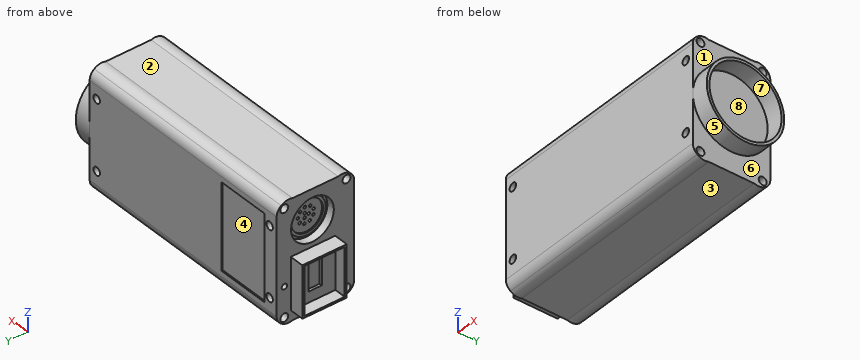
from build123d import *

# Parameters (mm, degrees)
SALIENTE_EXTRUIR2_DEPTH = 86.7
CROQUIS4_R              = 1.5
CORTAR_EXTRUIR1_DEPTH   = 4
CROQUIS5_R              = 14.5
CROQUIS5_R_2            = 13.5
SALIENTE_EXTRUIR3_DEPTH = 6.45
CROQUIS6_R              = 1.5
CORTAR_EXTRUIR2_DEPTH   = 3.5
CROQUIS8_W              = 20
CROQUIS8_H              = 32
CORTAR_EXTRUIR3_DEPTH   = 0.5
CROQUIS10_R             = 1
CORTAR_EXTRUIR6_DEPTH   = 4.5
CORTAR_EXTRUIR7_START   = -4.5
CROQUIS11_R             = 1.5
CORTAR_EXTRUIR7_DEPTH   = 4.5
CROQUIS12_W             = 19.288477202
CROQUIS12_H             = 16.6
SALIENTE_EXTRUIR4_DEPTH = 5.35
CROQUIS13_W             = 18
CROQUIS13_H             = 15.1
CORTAR_EXTRUIR8_DEPTH   = 4.35
CROQUIS14_W             = 10
CROQUIS14_H             = 5
CORTAR_EXTRUIR9_DEPTH   = 1
CROQUIS15_R             = 8
CORTAR_EXTRUIR10_DEPTH  = 3
CROQUIS16_R             = 7
CROQUIS16_R_2           = 6
SALIENTE_EXTRUIR5_DEPTH = 0.5
CROQUIS17_R             = 0.5
CORTAR_EXTRUIR12_DEPTH  = 1.5
CROQUIS18_R             = 1.5
CORTAR_EXTRUIR13_DEPTH  = 3.5


with BuildPart() as part:
    # Croquis3 → Saliente-Extruir2 (new body)
    with BuildSketch(Plane(origin=(0, 0, 0), x_dir=(0, 0, -1), z_dir=(1, 0, 0))):
        with BuildLine():
            Line((4, 0), (40, 0))
            ThreePointArc((40, 0), (41.842910618, 0.449833743), (43.271319545, 1.698159773))
            ThreePointArc((43.271319545, 1.698159773), (44.186191252, 3.744879364), (44, 5.979019946))
            Line((44, 5.979019946), (44, 23.020980054))
            ThreePointArc((44, 23.020980054), (44.186191252, 25.255120636), (43.271319545, 27.301840227))
            ThreePointArc((43.271319545, 27.301840227), (41.842910618, 28.550166257), (40, 29))
            Line((40, 29), (4, 29))
            ThreePointArc((4, 29), (2.157089382, 28.550166257), (0.728680455, 27.301840227))
            ThreePointArc((0.728680455, 27.301840227), (-0.186191252, 25.255120636), (0, 23.020980054))
            Line((0, 23.020980054), (0, 5.979019946))
            ThreePointArc((0, 5.979019946), (-0.186191252, 3.744879364), (0.728680455, 1.698159773))
            ThreePointArc((0.728680455, 1.698159773), (2.157089382, 0.449833743), (4, 0))
        make_face()
    extrude(amount=SALIENTE_EXTRUIR2_DEPTH)

    # Croquis4 → Cortar-Extruir1 (cut)
    with BuildSketch(Plane(origin=(86.7, 0, 0), x_dir=(0, 0, -1), z_dir=(1, 0, 0))):
        with Locations((2.364340227, 26.150920114)):
            Circle(CROQUIS4_R)
        with Locations(Location((41.635659773, 26.150920114, 0), (0, 0, 180))):
            Circle(CROQUIS4_R)
        with Locations((41.635659773, 2.849079886)):
            Circle(CROQUIS4_R)
        with Locations(Location((2.364340227, 2.849079886, 0), (0, 0, 180))):
            Circle(CROQUIS4_R)
    extrude(amount=-CORTAR_EXTRUIR1_DEPTH, mode=Mode.SUBTRACT)

    # Croquis5 → Saliente-Extruir3 (add)
    with BuildSketch(Plane(origin=(86.7, 0, 0), x_dir=(0, 0, -1), z_dir=(1, 0, 0))):
        with Locations(Location((22, 14.5, 0), (0, 0, 270))):
            Circle(CROQUIS5_R)
        with Locations(Location((22, 14.5, 0), (0, 0, 180))):
            Circle(CROQUIS5_R_2, mode=Mode.SUBTRACT)
    extrude(amount=SALIENTE_EXTRUIR3_DEPTH)

    # Croquis6 → Cortar-Extruir2 (cut)
    with BuildSketch(Plane(origin=(0, 29, 0), x_dir=(1, 0, 0), z_dir=(0, 1, 0))):
        with Locations(Location((83.45, 35, 0), (0, 0, 270))):
            Circle(CROQUIS6_R)
        with Locations(Location((83.45, 9, 0), (0, 0, 270))):
            Circle(CROQUIS6_R)
        with Locations(Location((3.25, 9, 0), (0, 0, 90))):
            Circle(CROQUIS6_R)
        with Locations(Location((3.25, 35, 0), (0, 0, 90))):
            Circle(CROQUIS6_R)
    extrude(amount=-CORTAR_EXTRUIR2_DEPTH, mode=Mode.SUBTRACT)

    # Croquis8 → Cortar-Extruir3 (cut)
    with BuildSketch(Plane(origin=(0, 29, 0), x_dir=(1, 0, 0), z_dir=(0, 1, 0))):
        with Locations((15.654947335, 22)):
            Rectangle(CROQUIS8_W, CROQUIS8_H)
    extrude(amount=-CORTAR_EXTRUIR3_DEPTH, mode=Mode.SUBTRACT)

    # Croquis10 → Cortar-Extruir6 (cut)
    with BuildSketch(Plane.ZY):
        with Locations((-30.5, 6.1)):
            Circle(CROQUIS10_R)
        with Locations((-30.5, 26.1)):
            Circle(CROQUIS10_R)
    extrude(amount=-CORTAR_EXTRUIR6_DEPTH, mode=Mode.SUBTRACT)

    # Croquis11 → Cortar-Extruir7 (cut)
    with BuildSketch(Plane.ZY.offset(CORTAR_EXTRUIR7_START)):
        with Locations((-41.635659773, 26.150920114)):
            Circle(CROQUIS11_R)
        with Locations(Location((-41.635659773, 2.849079886, 0), (0, 0, 180))):
            Circle(CROQUIS11_R)
        with Locations((-2.364340227, 2.849079886)):
            Circle(CROQUIS11_R)
        with Locations(Location((-2.364340227, 26.150920114, 0), (0, 0, 180))):
            Circle(CROQUIS11_R)
    extrude(amount=CORTAR_EXTRUIR7_DEPTH, mode=Mode.SUBTRACT)

    # Croquis12 → Saliente-Extruir4 (add)
    with BuildSketch(Plane.ZY):
        with Locations((-30.5, 15.4)):
            Rectangle(CROQUIS12_W, CROQUIS12_H)
    extrude(amount=SALIENTE_EXTRUIR4_DEPTH)

    # Croquis13 → Cortar-Extruir8 (cut)
    with BuildSketch(Plane.ZY.offset(5.35)):
        with Locations((-30.489294878, 15.4)):
            Rectangle(CROQUIS13_W, CROQUIS13_H)
    extrude(amount=-CORTAR_EXTRUIR8_DEPTH, mode=Mode.SUBTRACT)

    # Croquis14 → Cortar-Extruir9 (cut)
    with BuildSketch(Plane.ZY.offset(1)):
        with Locations((-30.5, 15.4)):
            Rectangle(CROQUIS14_W, CROQUIS14_H)
    extrude(amount=-CORTAR_EXTRUIR9_DEPTH, mode=Mode.SUBTRACT)

    # Croquis15 → Cortar-Extruir10 (cut)
    with BuildSketch(Plane.ZY):
        with Locations((-11.119013901, 15.6)):
            Circle(CROQUIS15_R)
    extrude(amount=-CORTAR_EXTRUIR10_DEPTH, mode=Mode.SUBTRACT)

    # Croquis16 → Saliente-Extruir5 (add)
    with BuildSketch(Plane.ZY.offset(-3)):
        with Locations((-11.119013901, 15.6)):
            Circle(CROQUIS16_R)
        with Locations((-11.119013901, 15.6)):
            Circle(CROQUIS16_R_2, mode=Mode.SUBTRACT)
    extrude(amount=SALIENTE_EXTRUIR5_DEPTH)

    # Croquis17 → Cortar-Extruir12 (cut)
    with BuildSketch(Plane.ZY.offset(-3)):
        with Locations((-11.025814876, 18.6)):
            Circle(CROQUIS17_R)
        with Locations((-9.119256477, 17.838226151)):
            Circle(CROQUIS17_R)
        with Locations((-8.148406801, 16.029161411)):
            Circle(CROQUIS17_R)
        with Locations((-8.567537202, 14.019287277)):
            Circle(CROQUIS17_R)
        with Locations((-10.180531906, 12.749046194)):
            Circle(CROQUIS17_R)
        with Locations((-12.232652766, 12.812798081)):
            Circle(CROQUIS17_R)
        with Locations((-13.763689624, 14.180712723)):
            Circle(CROQUIS17_R)
        with Locations((-14.057253319, 16.212727655)):
            Circle(CROQUIS17_R)
        with Locations((-12.975982135, 17.958040507)):
            Circle(CROQUIS17_R)
        with Locations((-11.985039305, 16.1)):
            Circle(CROQUIS17_R)
        with Locations((-10.252988497, 16.1)):
            Circle(CROQUIS17_R)
        with Locations((-11.119013901, 14.6)):
            Circle(CROQUIS17_R)
    extrude(amount=-CORTAR_EXTRUIR12_DEPTH, mode=Mode.SUBTRACT)

    # Croquis18 → Cortar-Extruir13 (cut)
    with BuildSketch(Plane.XZ):
        with Locations(Location((83.45, -8.377668185, 0), (0, 0, 270))):
            Circle(CROQUIS18_R)
        with Locations(Location((83.45, -34.377668185, 0), (0, 0, 270))):
            Circle(CROQUIS18_R)
        with Locations(Location((3.25, -34.377668185, 0), (0, 0, 90))):
            Circle(CROQUIS18_R)
        with Locations(Location((3.25, -8.377668185, 0), (0, 0, 90))):
            Circle(CROQUIS18_R)
    extrude(amount=-CORTAR_EXTRUIR13_DEPTH, mode=Mode.SUBTRACT)


solid = part.part
The listing builds one solid part. Answer for the finished solid, in the listing's coordinates (mm). Face numbers are marked on the shaded views. A direction names the side the tool comes from. Give positions to 0.01 mm unless a question says otherwise; leave off trailing zeros. Order: outer loops, then holes, each group sorted by start corner. A loop starts at its lowest first (then second) coordinate and runs counter-clockwise, first axis right, second up. Notation, with made-up numbers: (-25, 56.5) - (11, 56.5) arc R33 ccw to (11, 88.5) - close; hole circle Ø2 at (0, 48). An arc over 180 degrees is marked (long way). Answer as CSV lines item,"result".
Q1. A cutting plane is placed at A-A, the plane x = 74. Determine the outline of the cut face in (y, z), and give its area (3 significant figures).
Answer key:
outline,"(0, -40) arc R4 ccw to (1.7, -43.27) arc R4.5 ccw to (5.98, -44) - (23.02, -44) arc R4.5 ccw to (27.3, -43.27) arc R4 ccw to (29, -40) - (29, -4) arc R4 ccw to (27.3, -0.73) arc R4.5 ccw to (23.02, 0) - (5.98, 0) arc R4.5 ccw to (1.7, -0.73) arc R4 ccw to (0, -4) - close"
area,"1,260 mm^2"
Q2. Each of these flat-tipped pins is pushed along its axis until it touches: pin 1 Ø2.5 at (y, z) = (6.1, -30.5) entering from +X; pin 2 Ø0.6 at (y, z) = (6, -30.5) entering from -X; pin 3 Ø2.5 at (y, z) = (2.85, -2.36) entering from +X; pin 4 Ø5 at (x, z) = (-2, -34.5) entering from -Y. Where does it stop, or does it pass through?
Answer key:
pin 1,"stops at x = 86.7"
pin 2,"stops at x = 4.5"
pin 3,"stops at x = 82.7"
pin 4,"stops at y = 0"
Q3. Determine the mould class of the marked faces 5, 6, 7 and 8 for opening direction Z: pulls with the +Z half, pulls with the -Z half, needs draft (parallel to the pull), parting line crosses it, or undercut.
Answer key:
face 5,"parting line crosses it"
face 6,"needs draft"
face 7,"undercut"
face 8,"undercut"
Q4. Which of the six approach directions +Z, -Z, +X, -X, +Y, -Y give full straight-line access (tool end or side, diameter ignored) to the marked faces 1, 2, 3 and 4?
Answer key:
face 1,"+Z, +X"
face 2,"+Z, +X, -X"
face 3,"-Z, +X, -X"
face 4,"+Y"
Q5. Straight lines are drawn through the part: L1, parallel to X at y = 17.5, z = -30.5; L2, parallel to Z at x = 64, y = 7.5; L3, parallel to X at y = 14.5, z = -19. For each, find the intervals that lie inside material, in ascending order.
Answer key:
L1,"x = 0 to 86.7"
L2,"z = -44 to 0"
L3,"x = 3 to 86.7"
